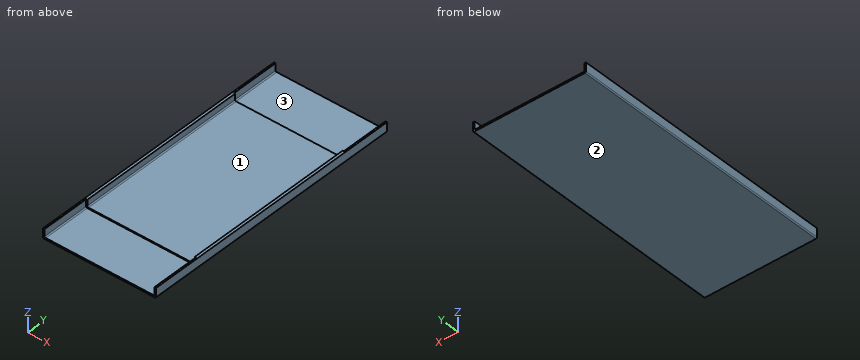
```python
from build123d import *

# Parameters (mm, degrees)
F1_DEPTH = 500
F2_DEPTH = 90


# Not quite as in the source:
# - a pattern or mirror of a feature is missing from the dataset's text; its kind, count and spacing are read off the source's solid


with BuildPart() as f1:
    # F0 (on Front) → F1 (new body)
    with BuildSketch(Plane.XZ):
        with BuildLine():
            Line((102, 0), (100, 0))
            Line((100, 0), (100, -11))
            ThreePointArc((100, -11), (99.4142135624, -12.4142135624), (98, -13))
            Line((98, -13), (0, -13))
            Line((0, -13), (-98, -13))
            ThreePointArc((-98, -13), (-99.4142135624, -12.4142135624), (-100, -11))
            Line((-100, -11), (-100, 0))
            Line((-100, 0), (-102, 0))
            Line((-102, 0), (-102, -13))
            ThreePointArc((-102, -13), (-101.4142135624, -14.4142135624), (-100, -15))
            Line((-100, -15), (100, -15))
            ThreePointArc((100, -15), (101.4142135624, -14.4142135624), (102, -13))
            Line((102, -13), (102, 0))
        make_face()
        with BuildLine():
            Line((105, 0), (102, 0))
            Line((102, 0), (102, -13))
            ThreePointArc((102, -13), (101.4142135624, -14.4142135624), (100, -15))
            Line((100, -15), (-100, -15))
            ThreePointArc((-100, -15), (-101.4142135624, -14.4142135624), (-102, -13))
            Line((-102, -13), (-102, 0))
            Line((-102, 0), (-105, 0))
            Line((-105, 0), (-105, -16))
            ThreePointArc((-105, -16), (-104.4142135624, -17.4142135624), (-103, -18))
            Line((-103, -18), (0, -18))
            Line((0, -18), (103, -18))
            ThreePointArc((103, -18), (104.4142135624, -17.4142135624), (105, -16))
            Line((105, -16), (105, 0))
        make_face()
    extrude(amount=F1_DEPTH)

    # F0 (on Front) → F2 (cut)
    with BuildSketch(Plane.XZ):
        with BuildLine():
            Line((102, 0), (100, 0))
            Line((100, 0), (100, -11))
            ThreePointArc((100, -11), (99.4142135624, -12.4142135624), (98, -13))
            Line((98, -13), (0, -13))
            Line((0, -13), (-98, -13))
            ThreePointArc((-98, -13), (-99.4142135624, -12.4142135624), (-100, -11))
            Line((-100, -11), (-100, 0))
            Line((-100, 0), (-102, 0))
            Line((-102, 0), (-102, -13))
            ThreePointArc((-102, -13), (-101.4142135624, -14.4142135624), (-100, -15))
            Line((-100, -15), (100, -15))
            ThreePointArc((100, -15), (101.4142135624, -14.4142135624), (102, -13))
            Line((102, -13), (102, 0))
        make_face()
    f2 = extrude(amount=F2_DEPTH, mode=Mode.SUBTRACT)

    # F2_copies: F2 across plane
    add(f2.mirror(Plane(origin=(0, -250, 0), x_dir=(0, 0, -1), z_dir=(0, -1, 0))), mode=Mode.SUBTRACT)


solid = f1.part
```
CAD build for the part. Positions are in the model's coordinates, mm. Face numbers are marked on the shaded views. Round coordinates to 2 decimals unless told otherwise and drop trailing zeros. Order: outer loops, then holes, each group sorted by start corner. A loop starts at its lowest first (then second) coordinate and runs counter-clockwise, first axis right, second up.
Q1. Slice it at D-D (y = -177). Write the cut outline in (x, z), and give its area (3 significant figures).
Q2. Wall check: L1, parallel to X at y = -369, z = -6; L2, parallel to X at y = -74.5, z = -8.75; L3, parallel to Z at x = -38, y = -131. Give the ranges that are in metal, low to high.
Q3. Slice it at C-C (x = -77). Write the cut outline in (y, z).
Q4. Drop flat-ended pins along their axis: pin 1 (7.5 mm diameter, centred on x = 5.5, z = -10.5, fed in from -Y); pin 2 (1.5 mm diameter, centred on x = 14.5, y = -404.5, fed in from +Z); pin 3 (6 mm diameter, centred on x = 31.5, y = -63, fed in from +Z). Give the stop position or say it passes through.
Q5. Slice it at B-B (y = -446.5). Write the cut outline in (x, z).
Q6. Slice it at A-A (z = -4.25). Write the cut outline in (x, y).
Q7. Two-plate mould, pull along X, no slides. Class the marked faces 1, 2 and 3: pulls with the +X half, pulls with the -X half, needs draft (parallel to the pull), parting line crosses it, or undercut.
Results below:
1. outline: (-105, -16) arc R2 ccw to (-103, -18) - (103, -18) arc R2 ccw to (105, -16) - (105, 0) - (100, 0) - (100, -11) arc R2 cw to (98, -13) - (-98, -13) arc R2 cw to (-100, -11) - (-100, 0) - (-105, 0) - close
1. area: 1,180 mm2
2. L1: x = -105 to -100, 100 to 105
2. L2: x = -105 to -102, 102 to 105
2. L3: z = -18 to -13
3. outline: (-500, -18) - (0, -18) - (0, -15) - (-90, -15) - (-90, -13) - (-410, -13) - (-410, -15) - (-500, -15) - close
4. pin 1: stops at y = -410
4. pin 2: stops at z = -13
4. pin 3: stops at z = -15
5. outline: (-105, -16) arc R2 ccw to (-103, -18) - (103, -18) arc R2 ccw to (105, -16) - (105, 0) - (102, 0) - (102, -13) arc R2 cw to (100, -15) - (-100, -15) arc R2 cw to (-102, -13) - (-102, 0) - (-105, 0) - close
6. outline: (-105, -500) - (-102, -500) - (-102, -410) - (-100, -410) - (-100, -90) - (-102, -90) - (-102, 0) - (-105, 0) - close; (100, -410) - (102, -410) - (102, -500) - (105, -500) - (105, 0) - (102, 0) - (102, -90) - (100, -90) - close
7. face 1: undercut
7. face 2: needs draft
7. face 3: undercut
